Part print with two shaded views. Sizes in mm from the minimum x, y, z corner. A direction names the side the tool comes from. Round coordinates to 2 decimals unless told otherwise and drop trailing zeros. Order: outer loops, then holes, each group sorted by start corner. A loop starts at its lowest first (then second) coordinate and runs counter-clockwise, first axis right, second up. Notation, with made-up numbers: (61, 81.25) -> (98, 81.25) arc R19 ccw to (98, 100.25) -> close; hole circle Ø1 at (-12.75, 25). An arc over 180 degrees is marked (long way). Put each result on its own line as item: value. Start each with the question number.
Q1. Cut at C-C, the plane x = 38. List the corners of the cut face in (y, z).
Q2. Pull direction Z, two halves, no side cores. Call the marked faces 3, 4 and 5: released by +Z, released by -Z, zero draft, split by the parting line, or undercut.
Q3. Flat gauge pins, fed straight in: P1, Ø6, axis at y = 13.5, z = 21, coming from the +X side; P2, Ø3, axis at y = 11, z = 28.5, coming from the +X side; P3, Ø3, axis at y = 7.5, z = 24, coming from the +X side. Where does each tip first touch, or does it go through?
Q4. Cut at D-D, the plane y = 20.25. List the corners of the cut face in (x, z).
Q5. 3-axis set-ups, long thin cutter, end or side, ignore diameter. For the marked faces 1 and 2: which of +Z, -Z, +X, -X, +Y, -Y reach the whole face in a straight line?
Q6. Cut at B-B, the plane y = 12.5. List the corners of the cut face in (x, z).
Q7. Probe L1, parallel to Z at x = 24.5, y = 14.5; L2, parallel to Y at x = 13, z = 1.5; L3, parallel to X at y = 7.75, z = 26. List the from-to ranges inside material, lowest first.
Q8. Cut at A-A, the plane x = 13. List the corners of the cut face in (y, z), and give its area (3 significant figures).
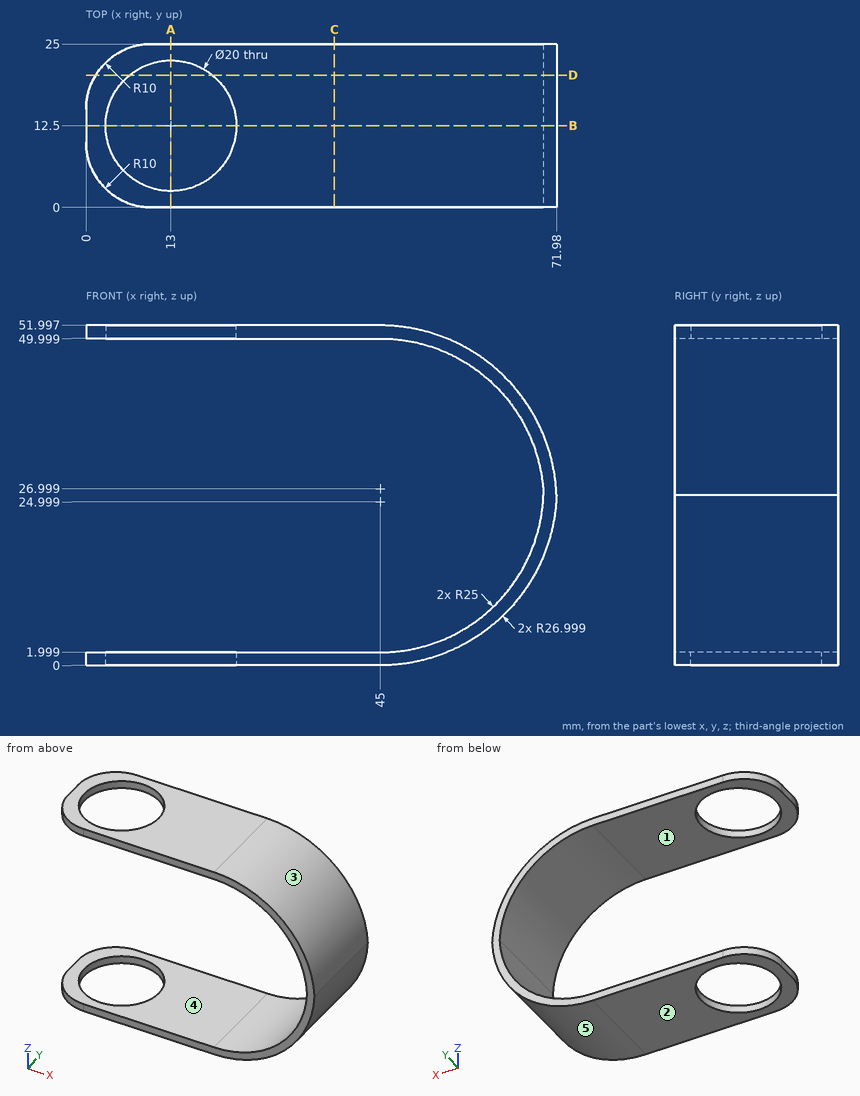
Ans:
1. outline: (0, 0) -> (25, 0) -> (25, 2) -> (0, 2) -> close; (0, 50) -> (25, 50) -> (25, 52) -> (0, 52) -> close
2. face 3: released by +Z
2. face 4: undercut
2. face 5: released by -Z
3. P1: stops at x = 71.83
3. P2: stops at x = 71.92
3. P3: stops at x = 71.96
4. outline: (1.49, 0) -> (6.68, 0) -> (6.68, 2) -> (1.49, 2) -> close; (1.49, 50) -> (6.68, 50) -> (6.68, 52) -> (1.49, 52) -> close; (19.32, 0) -> (45, 0) arc R27 ccw to (71.98, 26) arc R27 ccw to (45, 52) -> (19.32, 52) -> (19.32, 50) -> (45, 50) arc R25 cw to (69.98, 26) arc R25 cw to (45, 2) -> (19.32, 2) -> close
5. face 1: -X, +Y, -Y
5. face 2: -Z, +X, -X, +Y, -Y
6. outline: (0, 0) -> (3, 0) -> (3, 2) -> (0, 2) -> close; (0, 50) -> (3, 50) -> (3, 52) -> (0, 52) -> close; (23, 0) -> (45, 0) arc R27 ccw to (71.98, 26) arc R27 ccw to (45, 52) -> (23, 52) -> (23, 50) -> (45, 50) arc R25 cw to (69.98, 26) arc R25 cw to (45, 2) -> (23, 2) -> close
7. L1: z = 0 to 2, 50 to 52
7. L2: y = 0 to 2.5, 22.5 to 25
7. L3: x = 69.98 to 71.98
8. outline: (0, 0) -> (2.5, 0) -> (2.5, 2) -> (0, 2) -> close; (0, 50) -> (2.5, 50) -> (2.5, 52) -> (0, 52) -> close; (22.5, 0) -> (25, 0) -> (25, 2) -> (22.5, 2) -> close; (22.5, 50) -> (25, 50) -> (25, 52) -> (22.5, 52) -> close
8. area: 20.0 mm^2
